Here's how the part is built. I have some questions about the finished solid (model axes, mm). Face numbers are marked on the shaded views. Round coordinates to 2 decimals unless told otherwise and drop trailing zeros. Order: outer loops, then holes, each group sorted by start corner. A loop starts at its lowest first (then second) coordinate and runs counter-clockwise, first axis right, second up. Notation, with made-up numbers: (73, 67.25) -> (95, 67.25) arc R31 cw to (95, 106.25) -> close; hole circle Ø2 at (35.25, 12). An arc over 180 degrees is marked (long way). Use a Markdown table: item, result. Add a question column.
(1) I want a section at B-B, the plane z = 6.75. Please give me the cut outline in (x, y).
(2) I want a section at D-D, the plane x = 41.5. Please give me the cut outline in (y, z), then the cut area to 3 significant figures.
(3) I'm going to push flat-ended pins straight in: P1, Ø1.5, axis at x = 41.5, y = 70, coming from the -Z side; P2, Ø5, axis at y = 24.5, z = 5.5, coming from the +X side; P3, Ø4.5, axis at x = 48, y = 45, coming from the -Z side; P4, Ø2.5, axis at x = 48, y = 65, coming from the +Z side. Where does each tip first touch, or does it pass through?
(4) I want a section at C-C, the plane x = 47.5. Please give me the cut outline in (y, z).
(5) If I drill on probe 1 along Y at (x, z) = (48, 11.1); probe 2 along Y at (x, z) = (41.5, 9); probe 3 along X at (y, z) = (5, 11.5), over which ranges is the centre line in solid material (lowest first)?
(6) I want a section at A-A, the plane y = 45. Please give me the cut outline in (x, z).
(7) Thinking about a two-plate mould opening in Z: for the marked faces 1, 2 and 3, which applies, pulls with the +Z half, pulls with the -Z half, needs draft (parallel to the pull), parting line crosses it, or undercut?
Autodesk Inventor part; units mm, degrees
ref_plane "Right_Connecting_Web_StartPlane" through (0, 0, 4) normal (0, 0, 1) x (1, 0, 0)
ref_plane "Right_Rod_Contact_Flange_StartPlane" through (0, 0, 8.5) normal (0, 0, 1) x (1, 0, 0)
ref_plane "Work Plane3" through (0, 0, 4) normal (0, 0, 1) x (1, 0, 0)
ref_plane "Right_Connecting_Web_StartPlane" through (0, 0, 4) normal (0, 0, 1) x (1, 0, 0)
sketch "Right_Connecting_Web_Profile" plane through (0, 0, 4) normal (0, 0, 1) x (1, 0, 0)
  line L0 (39, 0) -> (45, 0)
  line L1 (45, 0) -> (45, 80)
  line L2 (45, 80) -> (39, 80)
  line L3 (39, 80) -> (39, 0)
  point P0 (0, 0)
  dimension "d1" = 39
  dimension "d2" = 6
  dimension "d3" = 80
extrude "Right_Connecting_Web" add sketch "Right_Connecting_Web_Profile" along normal blind 8.5
ref_plane "Right_Rod_Contact_Flange_StartPlane" through (0, 0, 8.5) normal (0, 0, 1) x (1, 0, 0)
sketch "Right_Rod_Contact_Flange_Profile" plane through (0, 0, 8.5) normal (0, 0, 1) x (1, 0, 0)
  line L0 (39, 0) -> (51, 0)
  line L1 (51, 0) -> (51, 80)
  line L2 (51, 80) -> (39, 80)
  line L3 (39, 80) -> (39, 0)
  point P0 (0, 0)
  dimension "d7" = 39
  dimension "d8" = 12
  dimension "d9" = 80
extrude "Right_Rod_Contact_Flange" add sketch "Right_Rod_Contact_Flange_Profile" along normal blind 4
sketch "Original_Rod_Clearance_4x_Locations" plane through (0, 0, 0) normal (0, 0, 1) x (1, 0, 0)
  circle A0 centre (48, 5) radius 1.7
  circle A1 centre (48, 25) radius 1.7
  circle A2 centre (48, 45) radius 1.7
  circle A3 centre (48, 65) radius 1.7
  point P0 (0, 0)
  dimension "d12" = 48
  dimension "d13" = 5
  dimension "d14" = 3.4
  dimension "d15" = 48
  dimension "d16" = 25
  dimension "d17" = 3.4
  dimension "d18" = 48
  dimension "d19" = 45
  dimension "d20" = 3.4
  dimension "d21" = 48
  dimension "d22" = 65
  dimension "d23" = 3.4
extrude "Original_Rod_Clearance_4x" cut sketch "Original_Rod_Clearance_4x_Locations" along normal through all
ref_plane "Work Plane3" through (0, 0, 4) normal (0, 0, 1) x (1, 0, 0)
sketch "Deck_Assembly_M3_Locations" plane through (0, 0, 4) normal (0, 0, 1) x (1, 0, 0)
  circle A0 centre (41.5, 10) radius 1.25
  circle A1 centre (41.5, 30) radius 1.25
  circle A2 centre (41.5, 50) radius 1.25
  circle A3 centre (41.5, 70) radius 1.25
  point P0 (0, 0)
  dimension "d27" = 41.5
  dimension "d28" = 10
  dimension "d29" = 2.5
  dimension "d30" = 41.5
  dimension "d31" = 30
  dimension "d32" = 2.5
  dimension "d33" = 41.5
  dimension "d34" = 50
  dimension "d35" = 2.5
  dimension "d36" = 41.5
  dimension "d37" = 70
  dimension "d38" = 2.5
extrude "Four_Blind_M3_Tap_Bores" cut sketch "Deck_Assembly_M3_Locations" along normal blind 6.5
thread "Deck_M3x0_5_6H_1"
thread "Deck_M3x0_5_6H_2"
thread "Deck_M3x0_5_6H_3"
thread "Deck_M3x0_5_6H_4"
equation "\"d2\" = WebThickness"
equation "\"d3\" = ContactLength"
equation "\"d4\" = DropHeight"
equation "\"d8\" = RodWidth + WebThickness"
equation "\"d9\" = ContactLength"
equation "\"d10\" = BaseThickness"
equation "\"d14\" = RodClearanceDiameter"
equation "\"d17\" = RodClearanceDiameter"
equation "\"d20\" = RodClearanceDiameter"
equation "\"d23\" = RodClearanceDiameter"
equation "\"d29\" = TapDrillDiameter"
equation "\"d32\" = TapDrillDiameter"
equation "\"d35\" = TapDrillDiameter"
equation "\"d38\" = TapDrillDiameter"
equation "\"d39\" = JoinThreadDepth"
equation "\"d41\" = JoinThreadDepth"
equation "\"d43\" = JoinThreadDepth"
equation "\"d45\" = JoinThreadDepth"
equation "\"d47\" = JoinThreadDepth"
equation "\"OverallWidth\" = 51"
equation "\"RodWidth\" = 6"
equation "\"ContactLength\" = 80"
equation "\"BaseThickness\" = 4"
equation "\"DropHeight\" = 8.5"
equation "\"WebThickness\" = 6"
equation "\"FingerStartX\" = 19.93338"
equation "\"FingerWidth\" = 13.5"
equation "\"FingerThickness\" = 6"
equation "\"FingerEndInset\" = 4"
equation "\"RodClearanceDiameter\" = 3.4"
equation "\"ClampFirstY\" = 41.82802"
equation "\"ClampPitch\" = 16"
equation "\"ClampHeight\" = BaseThickness + 0.5 * FingerThickness"
equation "\"TapDrillDiameter\" = 2.5"
equation "\"TapDepth\" = 6"
equation "\"RodHoleStart\" = 5"
equation "\"RodScrewPitch\" = 20"
equation "\"JoinLeftX\" = 9.5"
equation "\"JoinFirstY\" = 10"
equation "\"JoinPitch\" = 20"
equation "\"JoinThreadDepth\" = 6.5"
equation "\"JoinCountersinkDiameter\" = 6.2"
equation "\"d0\" = BaseThickness"
equation "\"d6\" = DropHeight"
equation "\"d26\" = BaseThickness"
properties part number "Right_Rod_Support"
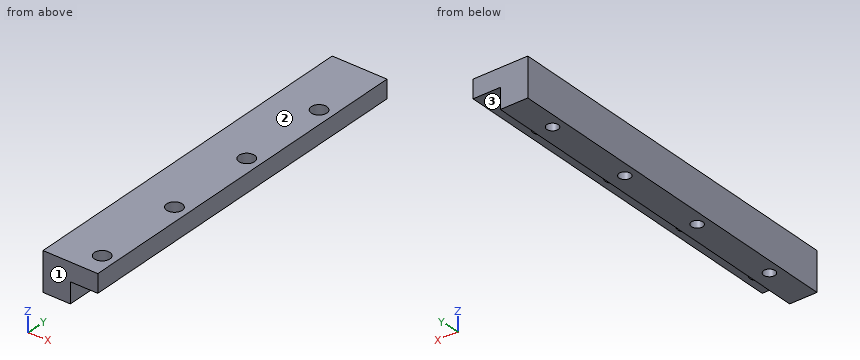
Taken from the geometry:
| question | item | result |
|---|---|---|
| 1 | outline | (39, 0) -> (45, 0) -> (45, 80) -> (39, 80) -> close; hole circle Ø2.5 at (41.5, 10); hole circle Ø2.5 at (41.5, 30); hole circle Ø2.5 at (41.5, 50); hole circle Ø2.5 at (41.5, 70) |
| 2 | outline | (0, 4) -> (8.75, 4) -> (8.75, 10.5) -> (11.25, 10.5) -> (11.25, 4) -> (28.75, 4) -> (28.75, 10.5) -> (31.25, 10.5) -> (31.25, 4) -> (48.75, 4) -> (48.75, 10.5) -> (51.25, 10.5) -> (51.25, 4) -> (68.75, 4) -> (68.75, 10.5) -> (71.25, 10.5) -> (71.25, 4) -> (80, 4) -> (80, 12.5) -> (0, 12.5) -> close |
| 2 | area | 615 mm2 |
| 3 | P1 | stops at z = 10.5 |
| 3 | P2 | stops at x = 45 |
| 3 | P3 | stops at z = 8.5 |
| 3 | P4 | passes through |
| 4 | outline | (0, 8.5) -> (3.38, 8.5) -> (3.38, 12.5) -> (0, 12.5) -> close; (6.62, 8.5) -> (23.38, 8.5) -> (23.38, 12.5) -> (6.62, 12.5) -> close; (26.62, 8.5) -> (43.38, 8.5) -> (43.38, 12.5) -> (26.62, 12.5) -> close; (46.62, 8.5) -> (63.38, 8.5) -> (63.38, 12.5) -> (46.62, 12.5) -> close; (66.62, 8.5) -> (80, 8.5) -> (80, 12.5) -> (66.62, 12.5) -> close |
| 5 | probe 1 | y = 0 to 3.3, 6.7 to 23.3, 26.7 to 43.3, 46.7 to 63.3, 66.7 to 80 |
| 5 | probe 2 | y = 0 to 8.75, 11.25 to 28.75, 31.25 to 48.75, 51.25 to 68.75, 71.25 to 80 |
| 5 | probe 3 | x = 39 to 46.3, 49.7 to 51 |
| 6 | outline | (39, 4) -> (45, 4) -> (45, 8.5) -> (46.3, 8.5) -> (46.3, 12.5) -> (39, 12.5) -> close; (49.7, 8.5) -> (51, 8.5) -> (51, 12.5) -> (49.7, 12.5) -> close |
| 7 | face 1 | needs draft |
| 7 | face 2 | pulls with the +Z half |
| 7 | face 3 | pulls with the -Z half |
